from build123d import *

# Parameters (mm, degrees)
BOSS_EXTRUDE1_DEPTH = 1.27


with BuildPart() as part:
    # Sketch1 → Boss-Extrude1 (new body)
    with BuildSketch(Plane(origin=(0, 0, 0), x_dir=(1, 0, 0), z_dir=(0, 1, 0))):
        with BuildLine():
            ThreePointArc((26.035, 33.655), (31.423153673, 31.423153673), (33.655, 26.035))
            add(Edge.make_bspline(
                [(33.655, 26.035), (36.449, 0), (33.655, -26.035)],
                knots=[0, 0, 0, 1, 1, 1], degree=2))
            ThreePointArc((33.655, -26.035), (31.423153673, -31.423153673), (26.035, -33.655))
            add(Edge.make_bspline(
                [(-26.035, -33.655), (0, -36.449), (26.035, -33.655)],
                knots=[0, 0, 0, 1, 1, 1], degree=2))
            ThreePointArc((-26.035, -33.655), (-31.423153673, -31.423153673), (-33.655, -26.035))
            add(Edge.make_bspline(
                [(-33.655, 26.035), (-36.449, 0), (-33.655, -26.035)],
                knots=[0, 0, 0, 1, 1, 1], degree=2))
            ThreePointArc((-33.655, 26.035), (-31.423153673, 31.423153673), (-26.035, 33.655))
            add(Edge.make_bspline(
                [(-26.035, 33.655), (0, 39.037083155), (26.035, 33.655)],
                knots=[0, 0, 0, 1, 1, 1], degree=2))
        make_face()
    extrude(amount=BOSS_EXTRUDE1_DEPTH)


solid = part.part
Geometry: final body of the model. Coordinates: model frame, mm. Give positions to 0.01 mm unless a question says otherwise; leave off trailing zeros. Write each loop counter-clockwise with the first axis right and the second up, starting at its lowest first coordinate (ties: lowest second). Pieces come first, ordered by that corner, then holes. Notation, with made-up numbers: (34, 52.25) -> (49, 52.25) arc R27 cw to (49, 73.25) -> close; hole circle Ø11 at (-40, 87.25). An arc over 180 degrees is marked (long way). Answer as a JSON object with one key per item and string values.
1. Ray query, probe 1 along Z at (x, y) = (1, 0.85); probe 2 along X at (y, z) = (1, -2); probe 3 along X at (y, z) = (0.8, 0). Return the intervals inside material, ascending. Write a range as from..to.
Ans:
{"probe 1": "z = -36.34..35.05", "probe 2": "x = -35.04..35.04", "probe 3": "x = -35.05..35.05"}
2. Cut plane B-B on x = 27.5. Output: boundary loops of the cut face in (y, z), and give its area (3 significant figures).
Ans:
{"outline": "(0, -33.51) -> (1.27, -33.51) -> (1.27, 33.51) -> (0, 33.51) -> close", "area": "85.1 mm^2"}
3. Cut plane A-A on z = -29. Output: boundary loops of the cut face in (x, y), and give its area (3 significant figures).
Ans:
{"outline": "(-33.05, 0) -> (33.05, 0) -> (33.05, 1.27) -> (-33.05, 1.27) -> close", "area": "84.0 mm^2"}
